Build history of the part. All positions in model axes, mm. Face numbers are marked on the shaded views. A direction names the side the tool comes from. Round coordinates to 2 decimals unless told otherwise and drop trailing zeros. Write each loop counter-clockwise with the first axis right and the second up, starting at its lowest first coordinate (ties: lowest second). Pieces come first, ordered by that corner, then holes. Notation, with made-up numbers: (62.25, 70) -> (69.25, 70) arc R18 cw to (69.25, 93) -> close; hole circle Ø1 at (33, -28.75). An arc over 180 degrees is marked (long way). Answer in a Markdown table with one row per item.
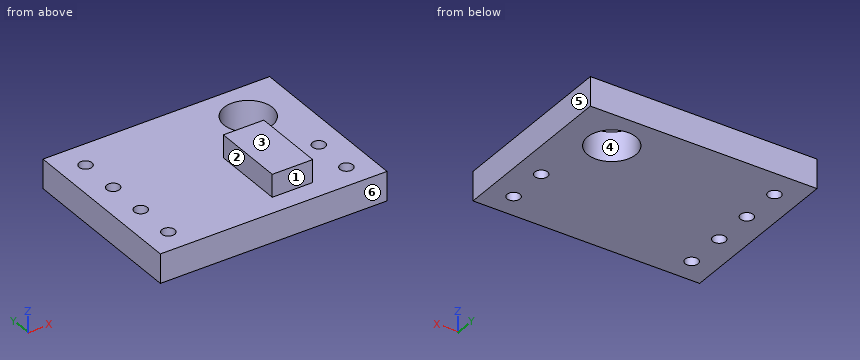
```python
from build123d import *

# Parameters (mm, degrees)
SKETCH_W     = 14
SKETCH_H     = 10.8
SKETCH_R     = 1.5
SKETCH_R_2   = 0.4
PAD_DEPTH    = 1.8
SKETCH001_W  = 2.5
SKETCH001_H  = 4.5
PAD001_DEPTH = 1.4


with BuildPart() as part:
    # Sketch → Pad (new body)
    with BuildSketch(Plane.XY):
        with Locations((-2, 1.9)):
            Rectangle(SKETCH_W, SKETCH_H)
        with Locations((2, 4.8)):
            Circle(SKETCH_R, mode=Mode.SUBTRACT)
        with Locations((3.5, 0.54)):
            Circle(SKETCH_R_2, mode=Mode.SUBTRACT)
        with Locations((3.5, -2)):
            Circle(SKETCH_R_2, mode=Mode.SUBTRACT)
        with Locations((-7.5, 5.62)):
            Circle(SKETCH_R_2, mode=Mode.SUBTRACT)
        with Locations((-7.5, 3.08)):
            Circle(SKETCH_R_2, mode=Mode.SUBTRACT)
        with Locations((-7.5, 0.54)):
            Circle(SKETCH_R_2, mode=Mode.SUBTRACT)
        with Locations((-7.5, -2)):
            Circle(SKETCH_R_2, mode=Mode.SUBTRACT)
    extrude(amount=PAD_DEPTH)

    # Sketch001 (on Face13 of Pad) → Pad001 (join)
    with BuildSketch(Plane.XY.offset(1.8)):
        Rectangle(SKETCH001_W, SKETCH001_H)
    extrude(amount=PAD001_DEPTH)


solid = part.part
```
Q1. Drop flat-ended pins along their axis: P1, Ø2, axis at x = -7, y = -1.5, coming from the +Z side; P2, Ø0.7, axis at x = -0.5, z = 2.5, coming from the -Y side. Give the stop position or say it passes through.
A:
| item | result |
|---|---|
| P1 | z = 1.8 |
| P2 | y = -2.25 |
Q2. Saw through at D-D on x = 2. Write the cut outline in (y, z), plus the area to 3 significant figures.
A:
| item | result |
|---|---|
| outline | (-3.5, 0) -> (3.3, 0) -> (3.3, 1.8) -> (-3.5, 1.8) -> close; (6.3, 0) -> (7.3, 0) -> (7.3, 1.8) -> (6.3, 1.8) -> close |
| area | 14.0 mm² |
Q3. Saw through at B-B on x = -7.5. Write the cut outline in (y, z).
A:
| item | result |
|---|---|
| outline | (-3.5, 0) -> (-2.4, 0) -> (-2.4, 1.8) -> (-3.5, 1.8) -> close; (-1.6, 0) -> (0.14, 0) -> (0.14, 1.8) -> (-1.6, 1.8) -> close; (0.94, 0) -> (2.68, 0) -> (2.68, 1.8) -> (0.94, 1.8) -> close; (3.48, 0) -> (5.22, 0) -> (5.22, 1.8) -> (3.48, 1.8) -> close; (6.02, 0) -> (7.3, 0) -> (7.3, 1.8) -> (6.02, 1.8) -> close |
Q4. Two-plate mould, pull along Y, no slides. Class the marked faces 4, 5 and 6: released by +Y, released by -Y, zero draft, split by the parting line, or undercut.
A:
| item | result |
|---|---|
| face 4 | undercut |
| face 5 | zero draft |
| face 6 | released by -Y |
Q5. Which spindle directions (+Z, -Z, +X, -X, +Y, -Y) get a long thin tool onto all of the face, cutting with end or side? Do the marked faces 1, 2 and 3. Say none if no direction does.
A:
| item | result |
|---|---|
| face 1 | +Z, +X, -X, -Y |
| face 2 | +Z, -X, +Y, -Y |
| face 3 | +Z, +X, -X, +Y, -Y |
Q6. Saw through at C-C on y = 4.8. Write the cut outline in (x, z), plus the area to 3 significant figures.
A:
| item | result |
|---|---|
| outline | (-9, 0) -> (0.5, 0) -> (0.5, 1.8) -> (-9, 1.8) -> close; (3.5, 0) -> (5, 0) -> (5, 1.8) -> (3.5, 1.8) -> close |
| area | 19.8 mm² |
Q7. Wall check: line 1 (Y direction, x = -7.5, z = 0.85); line 2 (X direction, y = 5.5, z = 0.85); line 3 (X direction, y = 0.75, z = 1.1). Give the ranges that are in metal, low to high. Write a range as [from, to].
A:
| item | result |
|---|---|
| line 1 | [-3.5, -2.4], [-1.6, 0.14], [0.94, 2.68], [3.48, 5.22], [6.02, 7.3] |
| line 2 | [-9, -7.88], [-7.12, 0.67], [3.33, 5] |
| line 3 | [-9, -7.84], [-7.16, 3.16], [3.84, 5] |
Q8. Saw through at A-A on y = 0.54. Write the cut outline in (x, z), plus the area to 3 significant figures.
A:
| item | result |
|---|---|
| outline | (-9, 0) -> (-7.9, 0) -> (-7.9, 1.8) -> (-9, 1.8) -> close; (-7.1, 0) -> (3.1, 0) -> (3.1, 1.8) -> (1.25, 1.8) -> (1.25, 3.2) -> (-1.25, 3.2) -> (-1.25, 1.8) -> (-7.1, 1.8) -> close; (3.9, 0) -> (5, 0) -> (5, 1.8) -> (3.9, 1.8) -> close |
| area | 25.8 mm² |
